Part model, mm, in its own coordinate system. Face numbers are marked on the shaded views. A direction names the side the tool comes from. Round coordinates to 2 decimals unless told otherwise and drop trailing zeros. Write each loop counter-clockwise with the first axis right and the second up, starting at its lowest first coordinate (ties: lowest second). Pieces come first, ordered by that corner, then holes.
```python
from build123d import *

# Parameters (mm, degrees)
CYLINDER004_R          = 1.8
CYLINDER004_DEPTH      = 40
CYLINDER005_R          = 1.8
CYLINDER005_DEPTH      = 40
CYLINDER006_R          = 1.5
CYLINDER006_DEPTH      = 40
ARRAY002_Y_COUNT       = 2
ARRAY002_Y_PITCH       = 10
ARRAY003_Y_COUNT       = 2
ARRAY003_Y_PITCH       = 40
CYLINDER003_R          = 1.8
CYLINDER003_DEPTH      = 80
BOX010_W               = 4
BOX010_H               = 58.6
BOX010_DEPTH           = 14
BOX013_W               = 10
BOX013_H               = 10
BOX013_DEPTH           = 4
ARRAY004_Z_COUNT       = 2
ARRAY004_Z_PITCH       = 54.5
BOX014_W               = 10
BOX014_H               = 4
BOX014_DEPTH           = 10
ARRAY005_Y_COUNT       = 2
ARRAY005_Y_PITCH       = 54.5
BOX011_W               = 10
BOX011_H               = 17
BOX011_DEPTH           = 2
BOX011_PLACEMENT_ANGLE = 45
BOX009_W               = 14
BOX009_H               = 55.6
BOX009_DEPTH           = 55.6
BOX012_W               = 2
BOX012_H               = 64
BOX012_DEPTH           = 64
FILLET005_R            = 2
BOX008_W               = 14
BOX008_H               = 58.6
BOX008_DEPTH           = 58.6


with BuildPart() as vert_bottom_hole:
    # Cylinder004 → Cylinder004 (new body)
    with BuildSketch(Plane(origin=(5, 30, -12), x_dir=(1, 0, 0), z_dir=(0, 0, 1))):
        Circle(CYLINDER004_R)
    extrude(amount=CYLINDER004_DEPTH)


with BuildPart() as vert_top_hole:
    # Cylinder005 → Cylinder005 (new body)
    with BuildSketch(Plane(origin=(8, 30, 40), x_dir=(1, 0, 0), z_dir=(0, 0, 1))):
        Circle(CYLINDER005_R)
    extrude(amount=CYLINDER005_DEPTH)


with BuildPart() as wall_hole_array_array:
    # Cylinder006 → Cylinder006 (new body)
    with BuildSketch(Plane(origin=(0, 5, 10.5), x_dir=(0, 0, -1), z_dir=(1, 0, 0))):
        Circle(CYLINDER006_R)
    extrude(amount=CYLINDER006_DEPTH)

    # Array002 Y: wall hole array array ×2


with BuildPart() as wall_hole_array_array_1:
    add(wall_hole_array_array.part)
    with Locations(*[(0, i * ARRAY002_Y_PITCH, 0) for i in range(1, ARRAY002_Y_COUNT)]):
        add(wall_hole_array_array.part)

    # Array003 Y: wall hole array array ×2


with BuildPart() as wall_hole_array_array_2:
    add(wall_hole_array_array_1.part)
    with Locations(*[(0, i * ARRAY003_Y_PITCH, 0) for i in range(1, ARRAY003_Y_COUNT)]):
        add(wall_hole_array_array_1.part)


with BuildPart() as wall_hole_array_array_3:
    # Array003 placement: moved
    add(wall_hole_array_array_2.part.moved(Location((-10, 0, 0))))


with BuildPart() as around_wall_hole_fusion:
    # Cylinder003 → Cylinder003 (new body)
    with BuildSketch(Plane(origin=(8, 71, 30), x_dir=(1, 0, 0), z_dir=(0, -1, 0))):
        Circle(CYLINDER003_R)
    extrude(amount=CYLINDER003_DEPTH)

    # Fusion005: union vert bottom hole, vert top hole, wall hole array array
    add(vert_bottom_hole.part)
    add(vert_top_hole.part)
    add(wall_hole_array_array_3.part)


with BuildPart() as bottom_addition:
    # Box010 → Box010 (new body)
    with BuildSketch(Plane(origin=(9, 0.5, 0.5), x_dir=(1, 0, 0), z_dir=(0, 0, 1))):
        with Locations((2, 29.3)):
            Rectangle(BOX010_W, BOX010_H)
    extrude(amount=BOX010_DEPTH)


with BuildPart() as obj1:
    # Box013 → Box013 (new body)
    with BuildSketch(Plane(origin=(2, 25, 0.5), x_dir=(1, 0, 0), z_dir=(0, 0, 1))):
        with Locations((5, 5)):
            Rectangle(BOX013_W, BOX013_H)
    extrude(amount=BOX013_DEPTH)

    # Array004 Z: obj1 ×2


with BuildPart() as obj1_1:
    add(obj1.part)
    with Locations(*[(0, 0, i * ARRAY004_Z_PITCH) for i in range(1, ARRAY004_Z_COUNT)]):
        add(obj1.part)


with BuildPart() as obj2:
    # Box014 → Box014 (new body)
    with BuildSketch(Plane(origin=(3, 0.5, 25), x_dir=(1, 0, 0), z_dir=(0, 0, 1))):
        with Locations((5, 2)):
            Rectangle(BOX014_W, BOX014_H)
    extrude(amount=BOX014_DEPTH)

    # Array005 Y: obj2 ×2


with BuildPart() as obj2_1:
    add(obj2.part)
    with Locations(*[(0, i * ARRAY005_Y_PITCH, 0) for i in range(1, ARRAY005_Y_COUNT)]):
        add(obj2.part)


with BuildPart() as camera_cable_hole:
    # Box011 → Box011 (new body)
    with BuildSketch(Plane.XY):
        with Locations((5, 8.5)):
            Rectangle(BOX011_W, BOX011_H)
    extrude(amount=BOX011_DEPTH)


with BuildPart() as camera_cable_hole_1:
    # Box011 placement: moved
    add(camera_cable_hole.part.moved(Location((8.41288, 20, 46.52))).rotate(Axis((8.41288, 20, 46.52), (0, 1, 0)), BOX011_PLACEMENT_ANGLE))


with BuildPart() as back_wall_hole_fusion:
    # Box009 → Box009 (new body)
    with BuildSketch(Plane(origin=(-2, 2, 2), x_dir=(1, 0, 0), z_dir=(0, 0, 1))):
        with Locations((7, 27.8)):
            Rectangle(BOX009_W, BOX009_H)
    extrude(amount=BOX009_DEPTH)

    # Fusion002: union camera cable hole
    add(camera_cable_hole_1.part)


with BuildPart() as back_back_wall_fillet:
    # Box012 → Box012 (new body)
    with BuildSketch(Plane(origin=(14, -2, -2), x_dir=(1, 0, 0), z_dir=(0, 0, 1))):
        with Locations((1, 32)):
            Rectangle(BOX012_W, BOX012_H)
    extrude(amount=BOX012_DEPTH)

    # Fillet005
    fillet005_edges = [back_back_wall_fillet.edges().sort_by_distance(p)[0] for p in [
        (15, -2, -2),
        (15, -2, 62),
        (15, 62, -2),
        (15, 62, 62),
    ]]
    fillet(fillet005_edges, radius=FILLET005_R)


with BuildPart() as back_wall_whole_cut:
    # Box008 → Box008 (new body)
    with BuildSketch(Plane(origin=(0, 0.5, 0.5), x_dir=(1, 0, 0), z_dir=(0, 0, 1))):
        with Locations((7, 29.3)):
            Rectangle(BOX008_W, BOX008_H)
    extrude(amount=BOX008_DEPTH)

    # Fusion004: union back back wall fillet
    add(back_back_wall_fillet.part)

    # Cut004002: cut back wall hole fusion
    add(back_wall_hole_fusion.part, mode=Mode.SUBTRACT)

    # Fusion003: union bottom addition, obj1, obj2
    add(bottom_addition.part)
    add(obj1_1.part)
    add(obj2_1.part)

    # Cut004003: cut around wall hole fusion
    add(around_wall_hole_fusion.part, mode=Mode.SUBTRACT)


solid = back_wall_whole_cut.part
```
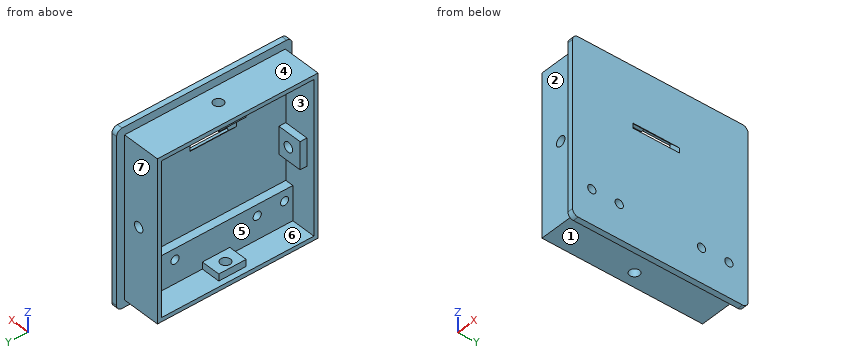
Q1. Wall check: L1, parallel to Y at x = 10.75, z = 10.5; L2, parallel to Z at x = 10.75, y = 5; L3, parallel to Z at x = 10.25, y = 37. Give the ranges that are in metal, low to high.
Values follow:
L1: y = 0.5 to 3.5, 6.5 to 13.5, 16.5 to 43.5, 46.5 to 53.5, 56.5 to 59.1
L2: z = 0.5 to 9, 12 to 14.5, 57.6 to 59.1
L3: z = 0.5 to 14.5, 57.6 to 59.1
Q2. Cut at A-A on y = 30. State how many separate pieces and enclosed holes the cut face has, plus the area to 3 significant figures.
Values follow:
separate pieces: 4
enclosed holes: 0
area: 322 mm2
Q3. Drop flat-ended pins along their axis: pin 1 (0.8 mm diameter, centred on y = 56.5, z = 28.5, fed in from -X); pin 2 (1.3 mm diameter, centred on x = 9, y = 56, fed in from -Z); pin 3 (8 mm diameter, centred on y = 29, z = 40.5, fed in from -X). Give the stop position or say it passes through.
Values follow:
pin 1: stops at x = 3
pin 2: stops at z = 0.5
pin 3: stops at x = 12
Q4. Mould opens along Z. For the marked faces 4, 5, 6 and 7 say: +Z half, -Z half, draft (parallel to the pull), parting line (faces both ways), or undercut.
Values follow:
face 4: +Z half
face 5: undercut
face 6: undercut
face 7: draft
Q5. Which spindle directions (+Z, -Z, +X, -X, +Y, -Y) get a long thin tool onto all of the face, cutting with end or side? Do the marked faces 1, 2 and 3. Say none if no direction does.
Values follow:
face 1: -Z, -X, +Y, -Y
face 2: +Z, -Z, -X, -Y
face 3: -X
Q6. Cut at B-B on z = 33. Write the cut outline in (x, y).
Values follow:
outline: (0, 0.5) - (14, 0.5) - (14, -2) - (16, -2) - (16, 62) - (14, 62) - (14, 59.1) - (0, 59.1) - (0, 57.6) - (3, 57.6) - (3, 55) - (12, 55) - (12, 4.5) - (3, 4.5) - (3, 2) - (0, 2) - close
Q7. Cut at D-D on y = 48. Write the cut outline in (x, z).
Values follow:
outline: (0, 0.5) - (14, 0.5) - (14, -2) - (16, -2) - (16, 62) - (14, 62) - (14, 59.1) - (0, 59.1) - (0, 57.6) - (12, 57.6) - (12, 14.5) - (9, 14.5) - (9, 2) - (0, 2) - close
